```python
from build123d import *

# Parameters (mm, degrees)
SKETCH_1_W          = 80
SKETCH_1_H          = 18
EXTRUDE_1_DEPTH     = 7
SKETCH_2_R          = 3.25
CUT_EXTRUDE_1_DEPTH = 5
SKETCH_3_R          = 1.75
CUT_EXTRUDE_3_DEPTH = 8


with BuildPart() as part:
    # 草图1 → 凸台-拉伸1 (new body)
    with BuildSketch(Plane(origin=(0, 0, 0), x_dir=(1, 0, 0), z_dir=(0, 1, 0))):
        with Locations((40, -9)):
            Rectangle(SKETCH_1_W, SKETCH_1_H)
    extrude(amount=EXTRUDE_1_DEPTH)

    # 草图2 → 切除-拉伸1 (cut)
    with BuildSketch(Plane(origin=(0, 7, 0), x_dir=(1, 0, 0), z_dir=(0, 1, 0))):
        with Locations((9.75, -9)):
            Circle(SKETCH_2_R)
        with Locations((39.75, -9)):
            Circle(SKETCH_2_R)
        with Locations((69.75, -9)):
            Circle(SKETCH_2_R)
    extrude(amount=-CUT_EXTRUDE_1_DEPTH, mode=Mode.SUBTRACT)

    # 草图3 → 切除-拉伸3 (cut, through all)
    with BuildSketch(Plane.XZ):
        with Locations((9.75, 9)):
            Circle(SKETCH_3_R)
        with Locations((39.75, 9)):
            Circle(SKETCH_3_R)
        with Locations((69.75, 9)):
            Circle(SKETCH_3_R)
    extrude(amount=-CUT_EXTRUDE_3_DEPTH, mode=Mode.SUBTRACT)


solid = part.part
```
Verification items for the finished model (mm, model axes). A direction names the side the tool comes from. Round coordinates to 2 decimals unless told otherwise and drop trailing zeros. Write each loop counter-clockwise with the first axis right and the second up, starting at its lowest first coordinate (ties: lowest second). Pieces come first, ordered by that corner, then holes. Notation, with made-up numbers: (5.25, 32.25) -> (51.25, 32.25) arc R20 cw to (51.25, 40.25) -> close; hole circle Ø10 at (26.5, -21.5). An arc over 180 degrees is marked (long way). Write each question's results on one line, items separated by ' | '. Start each with the question number.
1. Cross-section at B-B (x = 39.75). Enter the section's corners in (y, z), then the cut area to 3 significant figures.
2. Cross-section at D-D (y = 1). Enter the section's corners in (x, z).
3. Draft check along X on faces 3 (the cylindrical face through (71.419, 0.986, 9.526)), 4 (the flat face through (39, 3, 0)), 5 (the flat face through (0, 3, 9)). Enter one of: +X half, -X half, draft (parallel to the pull), parting line (faces both ways), or undercut.
4. Depth check by flat-ended pin: P1, Ø6, axis at x = 69.75, z = 9, coming from the +Y side; P2, Ø2, axis at x = 69.75, z = 9, coming from the +Y side. Enter the tip coordinate at first touch or a pass-through.
5. Cross-section at C-C (z = 9). Enter the section's corners in (x, y).
6. Set-up check for faces 1 (the flat face through (11.1, 2, 10.4)), 2 (the cylindrical face through (10.691, 0.986, 10.476)): record each of +Z, -Z, +X, -X, +Y, -Y from which the full face is reachable in a straight line by a thin tool's end or side.
7. Material ranges on probe 1 along X at (y, z) = (4.75, 9); probe 2 along Z at (x, y) = (69.75, 1.25); probe 3 along X at (y, z) = (4.75, 9.75), recorded low to high. Write a range as from..to.
8. Cross-section at A-A (y = 4). Enter the section's corners in (x, z), then the cut area to 3 significant figures.
Solutions:
1) outline: (0, 0) -> (7, 0) -> (7, 5.75) -> (2, 5.75) -> (2, 7.25) -> (0, 7.25) -> close; (0, 10.75) -> (2, 10.75) -> (2, 12.25) -> (7, 12.25) -> (7, 18) -> (0, 18) -> close | area: 86.5 mm2
2) outline: (0, 0) -> (80, 0) -> (80, 18) -> (0, 18) -> close; hole circle Ø3.5 at (9.75, 9); hole circle Ø3.5 at (39.75, 9); hole circle Ø3.5 at (69.75, 9)
3) face 3: undercut | face 4: draft | face 5: -X half
4) P1: stops at y = 2 | P2: passes through
5) outline: (0, 0) -> (8, 0) -> (8, 2) -> (6.5, 2) -> (6.5, 7) -> (0, 7) -> close; (11.5, 0) -> (38, 0) -> (38, 2) -> (36.5, 2) -> (36.5, 7) -> (13, 7) -> (13, 2) -> (11.5, 2) -> close; (41.5, 0) -> (68, 0) -> (68, 2) -> (66.5, 2) -> (66.5, 7) -> (43, 7) -> (43, 2) -> (41.5, 2) -> close; (71.5, 0) -> (80, 0) -> (80, 7) -> (73, 7) -> (73, 2) -> (71.5, 2) -> close
6) face 1: +Y | face 2: +Y, -Y
7) probe 1: x = 0..6.5, 13..36.5, 43..66.5, 73..80 | probe 2: z = 0..7.25, 10.75..18 | probe 3: x = 0..6.59, 12.91..36.59, 42.91..66.59, 72.91..80
8) outline: (0, 0) -> (80, 0) -> (80, 18) -> (0, 18) -> close; hole circle Ø6.5 at (9.75, 9); hole circle Ø6.5 at (39.75, 9); hole circle Ø6.5 at (69.75, 9) | area: 1,340 mm2
